Design review of the part built by this model. Coordinates are the model's own, in mm. A direction names the side the tool comes from. Round coordinates to 2 decimals unless told otherwise and drop trailing zeros. Loops run counter-clockwise (first coordinate to the right, second up) from the corner with the lowest first, then second, coordinate; pieces in that order, holes last. Notation, with made-up numbers: (-12.5, 55.5) - (41.5, 55.5) arc R11 ccw to (41.5, 67.5) - close; hole circle Ø7 at (-30.5, 32.5). An arc over 180 degrees is marked (long way). Return JSON: item names as keys, results as strings. Group by question number.
(1) We need section D-D, the plane z = 10.75. Write out the cut boundary in (x, y), and give its area (3 significant figures).
(2) The part is to be moulded in two halves that separate along X. For faces 5 (the flat face through (3, 0, 0)), 6 (the cylindrical face through (-6.3, 1.6, 2.89)), 7 (the cylindrical face through (6.3, 0.97, -2.89)), say which applies: pulls with the +X half, pulls with the -X half, needs draft (parallel to the pull), parting line crosses it, or undercut.
(3) We need section A-A, the plane x = -7. Write out the cut boundary in (y, z), and give its area (3 significant figures).
(4) We need section B-B, the plane y = 4. Write out the cut boundary in (x, z), and give its area (3 significant figures).
(5) Clearance check with flat-ended pins moving along their axes: pin 1 (1 mm diameter, centred on x = -6.5, z = -7.5, fed in from -Y); pin 2 (4 mm diameter, centred on y = -2.5, z = 4, fed in from -X); pin 3 (1.5 mm diameter, centred on y = 4, z = 4.5, fed in from -X). State where each tip first meets the part, or that it passes through.
(6) We need section C-C, the plane z = 8. Write out the cut boundary in (x, y), and give its area (3 significant figures).
(7) For faces 1 (the flat face through (-1.728, -2.887, -0.184)), 2 (the cylindrical face through (6.3, 1.6, 2.87)), 3 (the flat face through (-0.901, -3.6, -5)), 4 (the cylindrical face through (-6.3, 0.97, -2.87)), list the 3-axis set-ups (+Z, -Z, +X, -X, +Y, -Y) from which the entire face can be reached by the end or side of a thin tool; tool diameter is ignored.
(8) Wall thickness on L1, parallel to Y at x = 0.5, z = 9.25; L2, parallel to X at y = -3.5, z = -8; L3, parallel to X at y = 1.5, z = -1: over which ranges is each line inside the solid? List them lowest first. Write a range as [from, to].
from build123d import *

# Parameters (mm, degrees)
F1_DEPTH  = 5.7
F3_DEPTH  = 18.44198
F4_R      = 0.685572
F4_R_2    = 0.6855
F5_DEPTH  = 15.48248
F7_DEPTH  = 25
F10_R     = 4.298757
F11_R     = 0.956545
F14_DEPTH = 25


with BuildPart() as f1:
    # F0 (on Front) → F1 (new body, symmetric)
    with BuildSketch(Plane.XZ):
        with BuildLine():
            ThreePointArc((-8.3, 10.199632), (-6.682161, 5.213445), (-6.13493, 0))
            ThreePointArc((-6.13493, 0), (-6.682161, -5.213445), (-8.3, -10.199632))
            ThreePointArc((-8.3, -10.199632), (-4.404392, -12.390473), (0, -13.15))
            ThreePointArc((0, -13.15), (4.404392, -12.390473), (8.3, -10.199632))
            ThreePointArc((8.3, -10.199632), (6.682161, -5.213445), (6.13493, 0))
            ThreePointArc((6.13493, 0), (6.682161, 5.213445), (8.3, 10.199632))
            ThreePointArc((8.3, 10.199632), (4.404392, 12.390473), (0, 13.15))
            ThreePointArc((0, 13.15), (-4.404392, 12.390473), (-8.3, 10.199632))
        make_face()
    extrude(amount=F1_DEPTH, both=True)

    # F2 (on Right) → F3 (cut, symmetric)
    with BuildSketch(Plane.YZ):
        Polygon((-5.998229, -14.557695), (0, 13.152902), (-5.998229, 13.152902), align=None)
    extrude(amount=F3_DEPTH, both=True, mode=Mode.SUBTRACT)

    # F4 (on Front) → F5 (cut, symmetric)
    with BuildSketch(Plane.XZ):
        with Locations((-6.507615, 4.309945)):
            Circle(F4_R)
        with Locations((-6.507615, -4.309945)):
            Circle(F4_R)
        with Locations((-6.176657, 1.446914)):
            Circle(F4_R_2)
        with Locations((-6.176657, -1.446914)):
            Circle(F4_R_2)
        with Locations((6.507615, 4.309945)):
            Circle(F4_R)
        with Locations((6.176657, 1.446914)):
            Circle(F4_R_2)
        with Locations((6.176657, -1.446914)):
            Circle(F4_R_2)
        with Locations((6.507615, -4.309945)):
            Circle(F4_R)
    extrude(amount=F5_DEPTH, both=True, mode=Mode.SUBTRACT)

    # F6 (on Front) → F7 (cut)
    with BuildSketch(Plane.XZ):
        with BuildLine():
            Line((4.558944, 0), (4.558944, 11.317))
            Line((4.558944, 11.317), (3.703271, 11.317))
            ThreePointArc((3.703271, 11.317), (2.664347, 10.278075), (1.625422, 11.317))
            Line((1.625422, 11.317), (-0.900685, 11.317))
            Line((-0.900685, 11.317), (-0.900685, 0))
            Line((-0.900685, 0), (-0.900685, -11.317))
            Line((-0.900685, -11.317), (1.625422, -11.317))
            ThreePointArc((1.625422, -11.317), (2.664347, -10.278075), (3.703271, -11.317))
            Line((3.703271, -11.317), (4.558944, -11.317))
            Line((4.558944, -11.317), (4.558944, 0))
        make_face()
    extrude(amount=F7_DEPTH, mode=Mode.SUBTRACT)

    # F10 (on offset) → F12 section 0
    with BuildSketch(Plane.XY.offset(-13.5)):
        with Locations((-2.386769, -0.51822)):
            Circle(F10_R)
    # F11 (on offset) → F12 section 1
    with BuildSketch(Plane.XY.offset(6.5)):
        with Locations((-1.16075, -0.51719)):
            Circle(F11_R)
    loft(mode=Mode.SUBTRACT)

    # F13 (on offset) → F14 (cut)
    with BuildSketch(Plane.XY.offset(6.5)):
        with BuildLine():
            Line((0, -5.757191), (0, -0.359881))
            ThreePointArc((0, -0.359881), (-1.185312, 0.695174), (-2.285457, -0.448411))
            Line((-2.285457, -0.448411), (-2.285457, -5.757191))
            Line((-2.285457, -5.757191), (0, -5.757191))
        make_face()
    extrude(amount=F14_DEPTH, mode=Mode.SUBTRACT)


solid = f1.part
Solutions:
{
 "1": {"outline": "(-7.57, -0.52) - (-2.29, -0.52) - (-2.29, -0.45) arc R1.14 cw to (-0.09, 0) - (1.79, 0) - (1.79, -0.52) - (3.53, -0.52) - (3.53, 0) - (4.56, 0) - (4.56, -0.52) - (7.57, -0.52) - (7.57, 5.7) - (-7.57, 5.7) - close", "area": "90.5 mm^2"},
 "2": {"face 5": "undercut", "face 6": "pulls with the -X half", "face 7": "pulls with the +X half"},
 "3": {"outline": "(-5.26, -11.13) - (5.7, -11.13) - (5.7, -6.53) - (-4.26, -6.53) - close; (-1.43, 6.53) - (5.7, 6.53) - (5.7, 11.13) - (-0.44, 11.13) - close", "area": "78.6 mm^2"},
 "4": {"outline": "(-8.3, -10.2) arc R13.15 ccw to (0, -13.15) arc R13.15 ccw to (8.3, -10.2) arc R25.11 cw to (6.63, -4.98) arc R0.69 cw (long way) to (6.4, -3.63) arc R25.11 cw to (6.23, -2.13) arc R0.69 cw (long way) to (6.15, -0.76) arc R25.11 cw to (6.13, 0) arc R25.11 cw to (6.15, 0.76) arc R0.69 cw (long way) to (6.23, 2.13) arc R25.11 cw to (6.4, 3.63) arc R0.69 cw (long way) to (6.63, 4.98) arc R25.11 cw to (8.3, 10.2) arc R13.15 ccw to (0, 13.15) arc R13.15 ccw to (-8.3, 10.2) arc R25.11 cw to (-6.63, 4.98) arc R0.69 cw (long way) to (-6.4, 3.63) arc R25.11 cw to (-6.23, 2.13) arc R0.69 cw (long way) to (-6.15, 0.76) arc R25.11 cw to (-6.13, 0) arc R25.11 cw to (-6.15, -0.76) arc R0.69 cw (long way) to (-6.23, -2.13) arc R25.11 cw to (-6.4, -3.63) arc R0.69 cw (long way) to (-6.63, -4.98) arc R25.11 cw to start", "area": "340 mm^2"},
 "5": {"pin 1": "y = -4.58", "pin 2": "x = -6.81", "pin 3": "x = -6.69"},
 "6": {"outline": "(-7.44, -1.12) - (-2.29, -1.12) - (-2.29, -0.45) arc R1.14 cw to (-0.09, 0) - (4.56, 0) - (4.56, -1.12) - (7.44, -1.12) - (7.44, 5.7) - (-7.44, 5.7) - close", "area": "92.8 mm^2"},
 "7": {"face 1": "+Z, +X, -X, -Y", "face 2": "+X, +Y, -Y", "face 3": "+Z, -Y", "face 4": "-X, +Y, -Y"},
 "8": {"L1": "[0, 5.7]", "L2": "[-7.44, -3.64], [4.56, 7.44]", "L3": "[-5.66, -2.52], [-0.72, 5.66]"}
}
